Autodesk Inventor part; units mm, degrees
ref_plane "Start plane" through (0, 0, 0) normal (0, 0, 1) x (1, 0, 0)
ref_plane "End plane" through (0, 0, 306.305284) normal (0, 0, 1) x (1, 0, 0)
ref_plane "Orientation Work Plane" through (-30, 30, 0) normal (0, 0, -1) x (-1, 0, 0)
ref_plane "Start plane" through (0, 0, 0) normal (0, 0, 1) x (1, 0, 0)
ref_plane "End plane" through (0, 0, 306.305284) normal (0, 0, 1) x (1, 0, 0)
sketch "Sketch" plane through (-30, 30, 0) normal (0, 0, -1) x (-1, 0, 0)
  line L0 (-30, -26) -> (-30, 26)
  line L1 (-26, 30) -> (26, 30)
  line L2 (30, 26) -> (30, -26)
  line L3 (26, -30) -> (-26, -30)
  arc A0 (-30, -26) -> (-26, -30) centre (-26, -26) ccw
  arc A1 (30, 26) -> (26, 30) centre (26, 26) ccw
  arc A2 (-26, 30) -> (-30, 26) centre (-26, 26) ccw
  arc A3 (26, -30) -> (30, -26) centre (26, -26) ccw
  arc A4 (-26, 28) -> (-28, 26) centre (-26, 26) ccw
  line L4 (-26, 28) -> (26, 28)
  arc A5 (28, 26) -> (26, 28) centre (26, 26) ccw
  line L5 (28, 26) -> (28, -26)
  arc A6 (26, -28) -> (28, -26) centre (26, -26) ccw
  line L6 (26, -28) -> (-26, -28)
  arc A7 (-28, -26) -> (-26, -28) centre (-26, -26) ccw
  line L7 (-28, -26) -> (-28, 26)
  line L8 (0, 37.102134) -> (0, -37.102134) construction
  line L9 (-23.102134, 0) -> (23.102134, 0) construction
  dimension "d7" = 4
  dimension "d9" = 60
  dimension "d11" = 60
  dimension "d12" = 2
  dimension "d15" = 30
  dimension "d16" = 30
sketch "Sketch3" plane through (0, 0, 0) normal (0, 0, 1) x (1, 0, 0)
  line L0 (0, 0) -> (10, 0)
ref_plane "Work Plane3" through (0, 0, 0) normal (0, -1, 0) x (1, 0, 0)
sketch "Sketch4" plane through (0, 0, 0) normal (0, -1, 0) x (1, 0, 0)
  line L0 (-2, 0) -> (12, 0)
  line L1 (-120.61347, 306.305284) -> (31.768912, 306.305284)
  dimension "d18" = 306.30528
ref_plane "Orientation Work Plane" through (-30, 30, 0) normal (0, 0, -1) x (-1, 0, 0)
sketch3d "Sweep Path"
  arc A0 (-40.889008, 0, 310.582854) -> (0, 0, 0) centre (-1200, 0, 0) ccw
sweep "Body" add profiles "Sketch" path "Sweep Path"
equation "\"d7\" = G_IR"
equation "\"d9\" = G_W"
equation "\"d11\" = G_H"
equation "\"d12\" = G_T"
equation "\"d15\" = 0.5 * d9"
equation "\"d16\" = 0.5 * d11"
equation "\"G_W\" = 60"
equation "\"G_H\" = 60"
equation "\"G_T\" = 2"
equation "\"G_IR\" = 4"
equation "\"G_L\" = d18"
equation "\"G_OFFSET_START\" = 0"
equation "\"G_OFFSET_END\" = 0"
equation "\"d14\" = G_OFFSET_END + B_L"
equation "\"B_L\" = 306.30528"
properties part number "ISO 4019 - 60x60x2 - 306.305" material "Steel, Mild"
Part model, mm, in its own coordinate system. A direction names the side the tool comes from. Coordinates: 2 decimals unless noted, no trailing zeros. Order: outer loops, then holes, each group sorted by start corner. A loop starts at its lowest first (then second) coordinate and runs counter-clockwise, first axis right, second up.
(1) Tool access for faces 4 (the face through (-12.54, 30.36, 158.55)), 5 (the face through (-9.98, 29.64, 154.45)), 6 (the face through (-67.5, 29.6, 147)), 7 (the face through (-46, 0, 154)), 8 (the face through (-45, 2, 154)): list every direction of +Z, -Z, +X, -X, +Y, -Y with a clear straight run to the whole face (end or side of a thin tool).
Check sheet entries:
face 4: -Z
face 5: +Z, +X, +Y, -Y
face 6: +Z
face 7: +Z, -Z, +X, -X, -Y
face 8: none
(2) Probe L1, parallel to Y at x = -22, z = 13; L2, parallel to X at y = 13, z = 126.5; L3, parallel to X at y = 15, z = 259. List the from-to ranges inside material, lowest first.
Check sheet entries:
L1: y = 0 to 2, 58 to 60
L2: x = -67.04 to -65.03, -8.7 to -6.69
L3: x = -89.81 to -87.76, -30.33 to -28.28
(3) Pull direction Y, two halves, no side cores. Call faces 1 (the face through (-70.027, 30.364, 150.871)), 2 (the face through (-45, 60, 154)), 3 (the face through (-46, 58, 154)): pulls with the +Y half, pulls with the -Y half, needs draft (parallel to the pull), parting line crosses it, or undercut.
Check sheet entries:
face 1: needs draft
face 2: pulls with the +Y half
face 3: undercut
(4) Pin check, flat tips, straight feed: pin 1 Ø5 at (y, z) = (44.5, 72.5) entering from -X; pin 2 Ø3 at (x, z) = (-26.5, 260) entering from +Y. Stop position of each tip, or through.
Check sheet entries:
pin 1: stops at x = -62.47
pin 2: passes through
(5) Slice it at A-A, the plane y = 29. Write the cut outline in (x, z).
Check sheet entries:
outline: (-98.84, 295.05) arc R1140 cw to (-60, 0) - (-58, 0) arc R1142 ccw to (-96.91, 295.57) - close; (-42.82, 310.07) arc R1198 cw to (-2, 0) - (0, 0) arc R1200 ccw to (-40.89, 310.58) - close
